Geometry: see drawing. Coordinates: mm, zero at the bounding-box minimum. Round coordinates to 2 decimals unless told otherwise and drop trailing zeros. Loops run counter-clockwise (first coordinate to the right, second up) from the corner with the lowest first, then second, coordinate; pieces in that order, holes last.
(1) Section B-B, the plane x = 107. Return the cut outline in (y, z), plus the area to 3 significant figures.
(2) First-contact query: pin 1 Ø1.6 at (x, z) = (173.5, 3) entering from -Y; pin 2 Ø3 at (y, z) = (212, 3.5) entering from -X. Flat tips, straight axial feed; report the tip coordinate or a pass-through.
(3) Material intervals for probe 1 along Y at (x, z) = (79.5, 4); probe 2 along X at (y, z) = (102, 4.1) (3 decimals); probe 3 along Y at (x, z) = (246, 5.35), sorted ascending.
(4) Section A-A, the plane x = 73. Return the cut outline in (y, z), plus the area to 3 significant figures.
(5) Section C-C, the plane z = 3.75. Count the separate pieces of the cut face and the enclosed holes in it, plus the area to 3 significant figures.
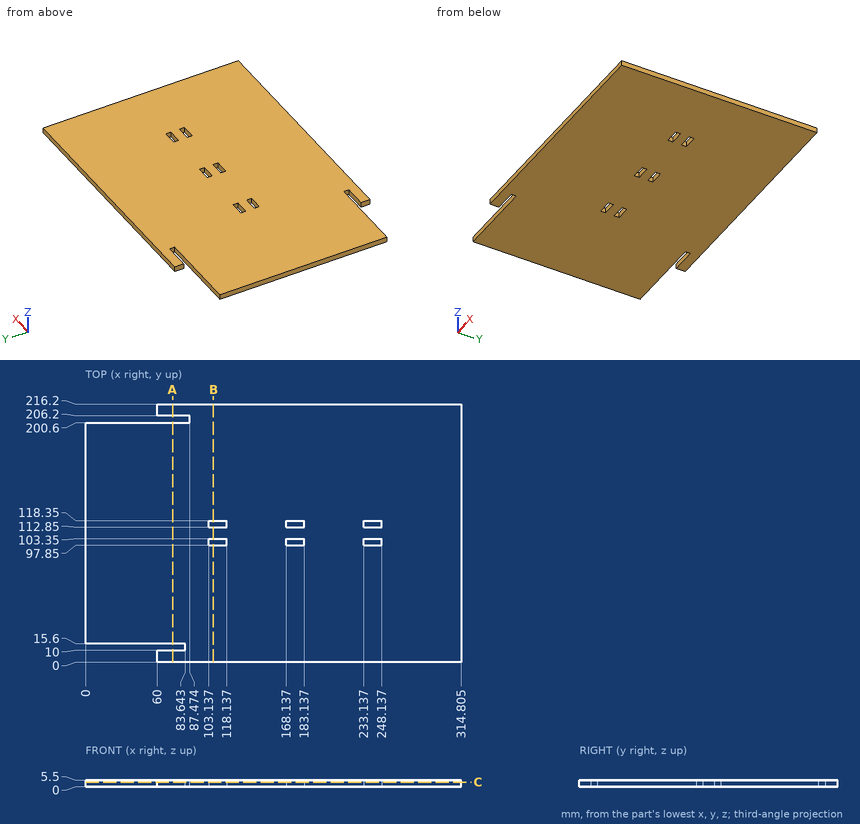
Output values:
1. outline: (0, 0) - (97.85, 0) - (97.85, 5.5) - (0, 5.5) - close; (103.35, 0) - (112.85, 0) - (112.85, 5.5) - (103.35, 5.5) - close; (118.35, 0) - (216.2, 0) - (216.2, 5.5) - (118.35, 5.5) - close
1. area: 1,130 mm2
2. pin 1: stops at y = 0
2. pin 2: stops at x = 60
3. probe 1: y = 0 to 10, 15.6 to 200.6, 206.2 to 216.2
3. probe 2: x = 0 to 103.137, 118.137 to 168.137, 183.137 to 233.137, 248.137 to 314.805
3. probe 3: y = 0 to 97.85, 103.35 to 112.85, 118.35 to 216.2
4. outline: (0, 0) - (10, 0) - (10, 5.5) - (0, 5.5) - close; (15.6, 0) - (200.6, 0) - (200.6, 5.5) - (15.6, 5.5) - close; (206.2, 0) - (216.2, 0) - (216.2, 5.5) - (206.2, 5.5) - close
4. area: 1,130 mm2
5. separate pieces: 1
5. enclosed holes: 6
5. area: 65,400 mm2
